Here's the drawing with two shaded views (mm, measured from the low corner). I have some questions. A direction names the side the tool comes from. Give positions to 0.01 mm unless a question says otherwise; leave off trailing zeros. Loops run counter-clockwise (first coordinate to the right, second up) from the corner with the lowest first, then second, coordinate; pieces in that order, holes last. Notation, with made-up numbers: (-24, -3) -> (-5, -3) arc R18 ccw to (-5, 1) -> close; hole circle Ø11 at (49.25, 87). An arc over 180 degrees is marked (long way). Answer in a Markdown table with one row per item. Add a question column.
Item 1: If I drill on line 1 (X direction, y = 1.75, z = 25.5); line 2 (X direction, y = 0.65, z = 6); line 3 (Y direction, x = 12.25, z = 15), over which ranges is the centre line in solid material (lowest first)?
Item 2: We'd pull the mould along X, two halves only. Please class the marked faces 3, 4 and 5: released by +X, released by -X, zero draft, split by the parting line, or undercut.
Item 3: For P1, Ø4, axis at x = 15.5, y = 5, coming from the -Z side; P2, Ø1.5, axis at x = 7, z = 8.5, coming from the +Y side; P3, Ø2.5, axis at x = 7.6, z = 21, coming from the -Y side, each with a flat end and sliding along its axis, tell me the tip position at first contact or that it passes through.
Item 4: If we section it at C-C (z = 6): Write out the boundary of the cut face in (x, y), then the cut area to 3 significant figures.
Item 5: If we section it at A-A (x = 7.6): Write out the boundary of the cut face in (y, z).
Item 6: Which directions (+Z, -Z, +X, -X, +Y, -Y) give clear straight access to the entire face, cutting with the end or side of a thin tool? Please do the marked faces 1 and 2.
Item 7: If we section it at D-D (x = 4): Write out the boundary of the cut face in (y, z), then the cut area to 3 significant figures.
Item 8: If we section it at B-B (y = 4.5): Write out the boundary of the cut face in (x, z).
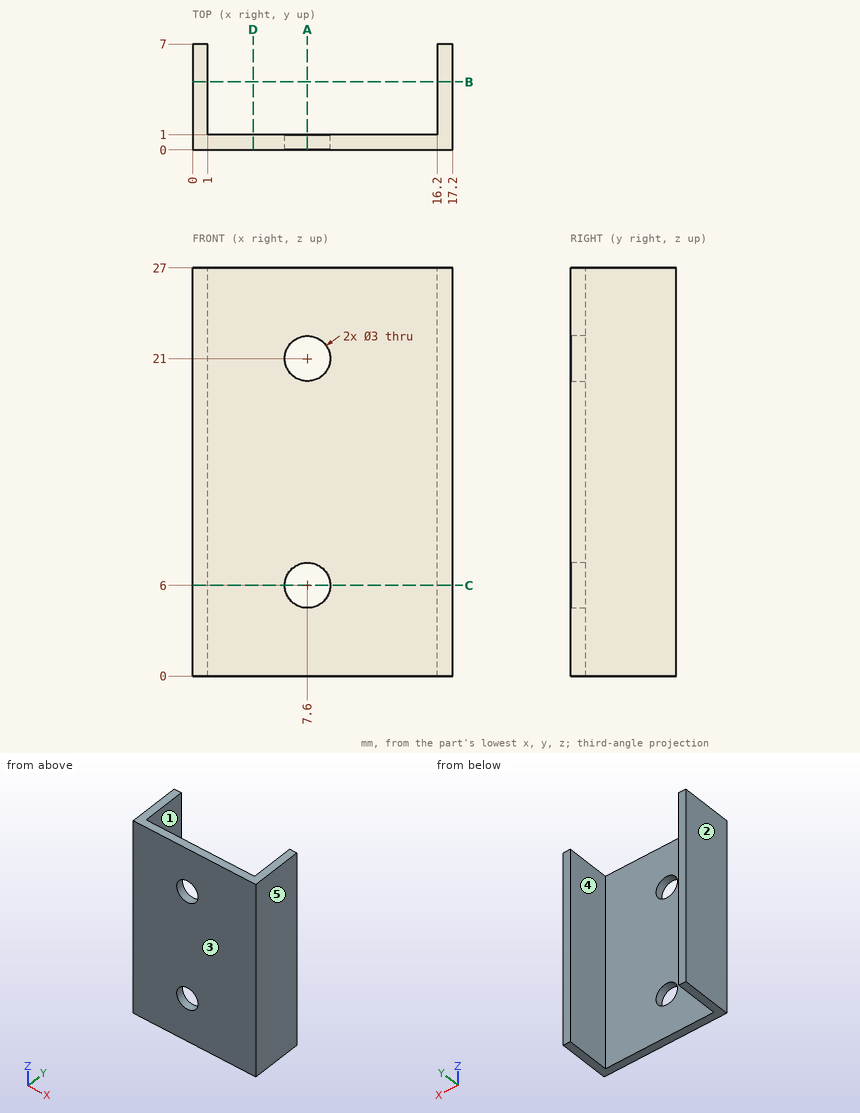
Recorded:
| question | item | result |
|---|---|---|
| 1 | line 1 | x = 0 to 1, 16.2 to 17.2 |
| 1 | line 2 | x = 0 to 6.1, 9.1 to 17.2 |
| 1 | line 3 | y = 0 to 1 |
| 2 | face 3 | zero draft |
| 2 | face 4 | undercut |
| 2 | face 5 | released by +X |
| 3 | P1 | stops at z = 0 |
| 3 | P2 | stops at y = 1 |
| 3 | P3 | passes through |
| 4 | outline | (0, 0) -> (6.1, 0) -> (6.1, 1) -> (1, 1) -> (1, 7) -> (0, 7) -> close; (9.1, 0) -> (17.2, 0) -> (17.2, 7) -> (16.2, 7) -> (16.2, 1) -> (9.1, 1) -> close |
| 4 | area | 26.2 mm^2 |
| 5 | outline | (0, 0) -> (1, 0) -> (1, 4.5) -> (0, 4.5) -> close; (0, 7.5) -> (1, 7.5) -> (1, 19.5) -> (0, 19.5) -> close; (0, 22.5) -> (1, 22.5) -> (1, 27) -> (0, 27) -> close |
| 6 | face 1 | +Z, -Z, +Y |
| 6 | face 2 | +Z, -Z, -X, +Y, -Y |
| 7 | outline | (0, 0) -> (1, 0) -> (1, 27) -> (0, 27) -> close |
| 7 | area | 27.0 mm^2 |
| 8 | outline | (0, 0) -> (1, 0) -> (1, 27) -> (0, 27) -> close; (16.2, 0) -> (17.2, 0) -> (17.2, 27) -> (16.2, 27) -> close |
